from build123d import *

# Parameters (mm, degrees)
SKETCH2_R           = 3.9
BOSS_EXTRUDE1_DEPTH = 5


with BuildPart() as part:
    # Sketch2 → Boss-Extrude1 (new body)
    with BuildSketch(Plane(origin=(0, 0, -1125.876159911), x_dir=(-1, 0, 0), z_dir=(0, 0, -1))):
        with BuildLine():
            Line((78, 17.5), (78, 32.5))
            Line((78, 32.5), (10.032697486, 93.651008078))
            ThreePointArc((10.032697486, 93.651008078), (0.028721986, 97.499972502), (-9.989920116, 93.689347438))
            Line((-9.989920116, 93.689347438), (-78, 32.969518252))
            Line((-78, 32.969518252), (-78, 17.5))
            Line((-78, 17.5), (-67.25, 17.5))
            Line((-67.25, 17.5), (-67.25, 23))
            ThreePointArc((-67.25, 23), (-62, 28.25), (-56.75, 23))
            Line((-56.75, 23), (-56.75, 17.5))
            Line((-56.75, 17.5), (56.75, 17.5))
            Line((56.75, 17.5), (56.75, 23))
            ThreePointArc((56.75, 23), (62, 28.25), (67.25, 23))
            Line((67.25, 23), (67.25, 17.5))
            Line((67.25, 17.5), (78, 17.5))
        make_face()
        with Locations((72, 22.5)):
            Circle(SKETCH2_R, mode=Mode.SUBTRACT)
        with Locations((-72, 22.5)):
            Circle(SKETCH2_R, mode=Mode.SUBTRACT)
    extrude(amount=BOSS_EXTRUDE1_DEPTH)


solid = part.part
Could you check a few things on this model? Use its own coordinates, in mm. A direction names the side the tool comes from. Coordinates: 2 decimals unless noted, no trailing zeros. Order: outer loops, then holes, each group sorted by start corner. A loop starts at its lowest first (then second) coordinate and runs counter-clockwise, first axis right, second up. Notation, with made-up numbers: (-27, 33.25) - (-7, 33.25) arc R15 cw to (-7, 39.25) - close; hole circle Ø7 at (-8, 54). An arc over 180 degrees is marked (long way). Answer in a Markdown table with one row per item. Add a question column.
(1) If we section it at D-D, the plane x = -62: Please give me the cut outline in (y, z), then the cut area to 3 significant figures.
(2) If we section it at B-B, the plane x = 72: Please give me the cut outline in (y, z).
(3) If we section it at C-C, the plane y = 74: Please give me the cut outline in (x, z), then the cut area to 3 significant figures.
(4) If we mould it in two halves opening along X, with no side actions, what happens to faces 3 (the face through (78, 25, -1128)), 4 (the face through (-0.2, 97.5, -1128.3)), 5 (the face through (-75.6, 21, -1128.3))? For each: released by +X, released by -X, zero draft, split by the parting line, or undercut.
(5) Will this pin go through, and if not, where does the flat tip stop? pin 1 (1.5 mm diameter, centred on x = -57.5, z = -1129.5, fed in from +Y).
(6) On a 3-axis mill with a long thin cutter (end or side, diameter ignored), from which of +Z, -Z, +X, -X, +Y, -Y can I reach the whole of each face in a straight line? I mean faces 1 (the face through (-56.75, 20, -1128)), 2 (the face through (68.4, 21, -1128.3)). Say none if no direction works.
(7) If we section it at A-A, the plane z = -1129.95: Please give me the cut outline in (x, y), then the cut area to 3 significant figures.
(8) I need wall thicknesses on L1, parallel to Y at x = 72, z = -1129.2; L2, parallel to Y at x = -71, z = -1129.2; L3, parallel to Y at x = 10, z = -1129. Which ranges of each line are inside material? Lowest first, please.
Results are:
| question | item | result |
|---|---|---|
| 1 | outline | (28.25, -1130.88) - (46.9, -1130.88) - (46.9, -1125.88) - (28.25, -1125.88) - close |
| 1 | area | 93.2 mm2 |
| 2 | outline | (17.5, -1130.88) - (18.6, -1130.88) - (18.6, -1125.88) - (17.5, -1125.88) - close; (26.4, -1130.88) - (38.33, -1130.88) - (38.33, -1125.88) - (26.4, -1125.88) - close |
| 3 | outline | (-31.87, -1130.88) - (32.04, -1130.88) - (32.04, -1125.88) - (-31.87, -1125.88) - close |
| 3 | area | 320 mm2 |
| 4 | face 3 | released by +X |
| 4 | face 4 | split by the parting line |
| 4 | face 5 | undercut |
| 5 | pin 1 | stops at y = 51.62 |
| 6 | face 1 | +Z, -Z, -Y |
| 6 | face 2 | +Z, -Z |
| 7 | outline | (-78, 17.5) - (-67.25, 17.5) - (-67.25, 23) arc R5.25 cw to (-56.75, 23) - (-56.75, 17.5) - (56.75, 17.5) - (56.75, 23) arc R5.25 cw to (67.25, 23) - (67.25, 17.5) - (78, 17.5) - (78, 32.97) - (9.99, 93.69) arc R15 ccw to (-10.03, 93.65) - (-78, 32.5) - close; hole circle Ø7.8 at (-72, 22.5); hole circle Ø7.8 at (72, 22.5) |
| 7 | area | 7,490 mm2 |
| 8 | L1 | y = 17.5 to 18.6, 26.4 to 38.33 |
| 8 | L2 | y = 17.5 to 18.73, 26.27 to 38.8 |
| 8 | L3 | y = 17.5 to 93.68 |
